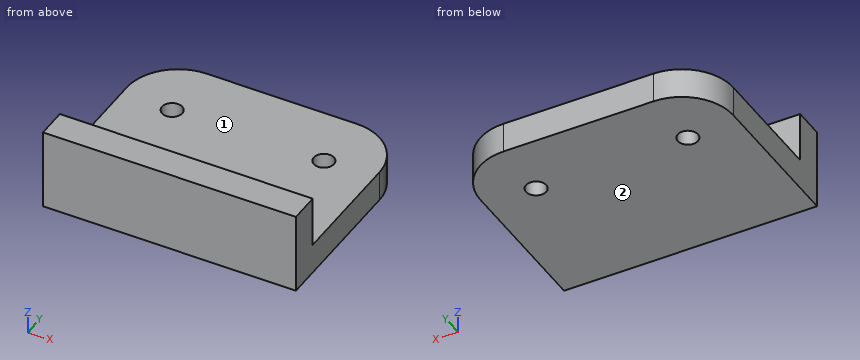
```python
from build123d import *

# Parameters (mm, degrees)
F0_R     = 1
F1_DEPTH = 3
F2_W     = 25
F2_H     = 3
F3_DEPTH = 5


with BuildPart() as f1:
    # F0 (on Top) → F1 (new body)
    with BuildSketch(Plane.XY):
        with BuildLine():
            Line((0, 14.92), (0, 0))
            Line((0, 0), (25, 0))
            Line((25, 0), (25, 14.92))
            ThreePointArc((25, 14.92), (23.512102, 18.512102), (19.92, 20))
            Line((19.92, 20), (5.08, 20))
            ThreePointArc((5.08, 20), (1.487898, 18.512102), (0, 14.92))
        make_face()
        with Locations((5, 14)):
            Circle(F0_R, mode=Mode.SUBTRACT)
        with Locations((20, 14)):
            Circle(F0_R, mode=Mode.SUBTRACT)
    extrude(amount=F1_DEPTH)

    # F2 (on face) → F3 (join)
    with BuildSketch(Plane.XY.offset(3)):
        with Locations((12.5, 1.5)):
            Rectangle(F2_W, F2_H)
    extrude(amount=F3_DEPTH)


solid = f1.part
```
CAD build for the part. Positions are in the model's coordinates, mm. Face numbers are marked on the shaded views. A direction names the side the tool comes from. Round coordinates to 2 decimals unless told otherwise and drop trailing zeros. Write each loop counter-clockwise with the first axis right and the second up, starting at its lowest first coordinate (ties: lowest second). Pieces come first, ordered by that corner, then holes. Notation, with made-up numbers: (18, 4.5) -> (70, 4.5) arc R11 cw to (70, 13.5) -> close; hole circle Ø6 at (84.5, -8). An arc over 180 degrees is marked (long way). Answer in a Markdown table with one row per item. Add a question column.
Item 1: Saw through at B-B, the plane x = 4.5. Write the cut outline in (y, z).
Item 2: Which spindle directions (+Z, -Z, +X, -X, +Y, -Y) get a long thin tool onto all of the face, cutting with end or side? Do the marked faces 1 and 2. Say none if no direction does.
Item 3: Saw through at A-A, the plane y = 14. Write the cut outline in (x, z), then the cut area to 3 significant figures.
Item 4: Saw through at D-D, the plane x = 8.5. Write the cut outline in (y, z), then the cut area to 3 significant figures.
Item 5: Drop flat-ended pins along their axis: pin 1 Ø1 at (x, z) = (17.5, 2.5) entering from -Y; pin 2 Ø2.5 at (x, y) = (20, 14) entering from +Z; pin 3 Ø4 at (x, z) = (6.5, 5.5) entering from +Y; pin 4 Ø4 at (y, z) = (7.5, 6.5) entering from +X. Give the stop position or say it passes through.
Item 6: Saw through at C-C, the plane z = 0.5. Write the cut outline in (x, y).
Item 7: Drill centre lines: line 1 (Y direction, x = 20, z = 1.2); line 2 (Y direction, x = 22.5, z = 5). Where is each one in solid material? Low to high. Write a range as from..to.
Findings below:
| question | item | result |
|---|---|---|
| 1 | outline | (0, 0) -> (13.13, 0) -> (13.13, 3) -> (3, 3) -> (3, 8) -> (0, 8) -> close; (14.87, 0) -> (19.97, 0) -> (19.97, 3) -> (14.87, 3) -> close |
| 2 | face 1 | +Z, +X, -X, +Y |
| 2 | face 2 | -Z, +X, -X, +Y, -Y |
| 3 | outline | (0, 0) -> (4, 0) -> (4, 3) -> (0, 3) -> close; (6, 0) -> (19, 0) -> (19, 3) -> (6, 3) -> close; (21, 0) -> (25, 0) -> (25, 3) -> (21, 3) -> close |
| 3 | area | 63.0 mm^2 |
| 4 | outline | (0, 0) -> (20, 0) -> (20, 3) -> (3, 3) -> (3, 8) -> (0, 8) -> close |
| 4 | area | 75.0 mm^2 |
| 5 | pin 1 | stops at y = 0 |
| 5 | pin 2 | stops at z = 3 |
| 5 | pin 3 | stops at y = 3 |
| 5 | pin 4 | passes through |
| 6 | outline | (0, 0) -> (25, 0) -> (25, 14.92) arc R5.08 ccw to (19.92, 20) -> (5.08, 20) arc R5.08 ccw to (0, 14.92) -> close; hole circle Ø2 at (5, 14); hole circle Ø2 at (20, 14) |
| 7 | line 1 | y = 0..13, 15..20 |
| 7 | line 2 | y = 0..3 |
